```python
from build123d import *

# Parameters (mm, degrees)
SKETCH_1_R      = 1.25
EXTRUDE_1_DEPTH = 2.8
SKETCH_2_R      = 4
SKETCH_2_R_2    = 1.25
EXTRUDE_2_DEPTH = 1.4
SKETCH_3_R      = 1.25
EXTRUDE_3_DEPTH = 2.8
EXTRUDE_4_DEPTH = 3


with BuildPart() as part:
    # 草图1 → 凸台-拉伸1 (new body)
    with BuildSketch(Plane(origin=(0, 0, 0), x_dir=(1, 0, 0), z_dir=(0, 1, 0))):
        with BuildLine():
            Line((0, 5.25), (9.5, 5.25))
            ThreePointArc((9.5, 5.25), (14.75, 0), (9.5, -5.25))
            Line((9.5, -5.25), (0, -5.25))
            ThreePointArc((0, -5.25), (-5.25, 0), (0, 5.25))
        make_face()
        Circle(SKETCH_1_R, mode=Mode.SUBTRACT)
        with Locations((9.5, 0)):
            Circle(SKETCH_1_R, mode=Mode.SUBTRACT)
    extrude(amount=EXTRUDE_1_DEPTH)

    # 草图2 → 凸台-拉伸2 (add)
    with BuildSketch(Plane(origin=(0, 2.8, 0), x_dir=(1, 0, 0), z_dir=(0, 1, 0))):
        Circle(SKETCH_2_R)
        Circle(SKETCH_2_R_2, mode=Mode.SUBTRACT)
        with Locations((9.5, 0)):
            Circle(SKETCH_2_R)
        with Locations((9.5, 0)):
            Circle(SKETCH_2_R_2, mode=Mode.SUBTRACT)
    extrude(amount=EXTRUDE_2_DEPTH)

    # 草图3 → 凸台-拉伸3 (add)
    with BuildSketch(Plane(origin=(0, 4.2, 0), x_dir=(1, 0, 0), z_dir=(0, 1, 0))):
        with BuildLine():
            Line((0, 5.25), (9.5, 5.25))
            ThreePointArc((9.5, 5.25), (14.75, 0), (9.5, -5.25))
            Line((9.5, -5.25), (0, -5.25))
            ThreePointArc((0, -5.25), (-5.25, 0), (0, 5.25))
        make_face()
        Circle(SKETCH_3_R, mode=Mode.SUBTRACT)
        with Locations((9.5, 0)):
            Circle(SKETCH_3_R, mode=Mode.SUBTRACT)
    extrude(amount=EXTRUDE_3_DEPTH)

    # 草图4 → 凸台-拉伸4 (add)
    with BuildSketch(Plane(origin=(0, 0, -5.25), x_dir=(-1, 0, 0), z_dir=(0, 0, -1))):
        with BuildLine():
            ThreePointArc((-1.932304569, 5.576196633), (-4.75, 7), (-7.567695431, 5.576196633))
            Line((-7.567695431, 5.576196633), (-6.360111675, 4.686398076))
            ThreePointArc((-6.360111675, 4.686398076), (-4.75, 5.5), (-3.139888325, 4.686398076))
            Line((-3.139888325, 4.686398076), (-1.932304569, 5.576196633))
        make_face()
        with BuildLine():
            Line((-6.360111675, 2.313601924), (-7.567695431, 1.423803367))
            ThreePointArc((-7.567695431, 1.423803367), (-4.75, 0), (-1.932304569, 1.423803367))
            Line((-1.932304569, 1.423803367), (-3.139888325, 2.313601924))
            ThreePointArc((-3.139888325, 2.313601924), (-4.75, 1.5), (-6.360111675, 2.313601924))
        make_face()
        with BuildLine():
            Line((-6.360111675, 4.686398076), (-7.567695431, 5.576196633))
            ThreePointArc((-7.567695431, 5.576196633), (-8.168041846, 4.252987343), (-8.17928564, 2.8))
            Line((-8.17928564, 2.8), (-6.6234994, 2.8))
            ThreePointArc((-6.6234994, 2.8), (-6.730785439, 3.77656653), (-6.360111675, 4.686398076))
        make_face()
        with BuildLine():
            ThreePointArc((-1.932304569, 1.423803367), (-1.551614092, 2.078617721), (-1.32071436, 2.8))
            Line((-1.32071436, 2.8), (-2.8765006, 2.8))
            ThreePointArc((-2.8765006, 2.8), (-2.99129812, 2.547651483), (-3.139888325, 2.313601924))
            Line((-3.139888325, 2.313601924), (-1.932304569, 1.423803367))
        make_face()
        with BuildLine():
            ThreePointArc((-1.25, 3.5), (-1.424948571, 4.592718169), (-1.932304569, 5.576196633))
            Line((-1.932304569, 5.576196633), (-3.139888325, 4.686398076))
            ThreePointArc((-3.139888325, 4.686398076), (-2.849970612, 4.124410382), (-2.75, 3.5))
            ThreePointArc((-2.75, 3.5), (-2.781879221, 3.144330771), (-2.8765006, 2.8))
            Line((-2.8765006, 2.8), (-1.32071436, 2.8))
            ThreePointArc((-1.32071436, 2.8), (-1.267723464, 3.148218633), (-1.25, 3.5))
        make_face()
        with BuildLine():
            Line((-6.6234994, 2.8), (-8.17928564, 2.8))
            ThreePointArc((-8.17928564, 2.8), (-7.948385908, 2.078617721), (-7.567695431, 1.423803367))
            Line((-7.567695431, 1.423803367), (-6.360111675, 2.313601924))
            ThreePointArc((-6.360111675, 2.313601924), (-6.50870188, 2.547651483), (-6.6234994, 2.8))
        make_face()
    extrude(amount=EXTRUDE_4_DEPTH)


solid = part.part
```
Geometry check sheet. Reference: the model listing, model coordinates, mm. A direction names the side the tool comes from. Coordinates: 2 decimals unless noted, no trailing zeros. Loops run counter-clockwise (first coordinate to the right, second up) from the corner with the lowest first, then second, coordinate; pieces in that order, holes last.
Item 1: Release check for a two-part mould opening along Y. For faces 6 (the face through (5.504, 3.49, -0.176)), 7 (the face through (5, 6, 5.25)), 8 (the face through (5, 7, 0)) record: released by +Y, released by -Y, zero draft, split by the parting line, or undercut.
Item 2: Thickness scan on line 1 (X direction, y = 2, z = 0); line 2 (X direction, y = 3.5, z = 0); line 3 (Y direction, x = 5, z = -4). Record the ranges inside material, lowest first.
Item 3: Access from +Z, -Z, +X, -X, +Y, -Y to the whole of each face (thin tool, end or side, straight path). Record for faces 1 (the face through (7, 4, -5.25)), 2 (the face through (-0.867, 3.49, 3.905)), 3 (the face through (5, 5, -5.25)), 4 (the face through (8, 6, -5.25)), 5 (the face through (1, 6, -5.25)).
Item 4: Sectioned sample at A-A, the plane z = 0. Record the boundary of the cut face in (x, y).
Item 5: Sectioned sample at C-C, the plane y = 3.25. Record the boundary of the cut face in (x, z), then the cut area to 3 significant figures.
Item 6: Go/stop test with flat-tipped pins: pin 1 Ø1 at (y, z) = (4, -2) entering from -X; pin 2 Ø2 at (y, z) = (3.5, 1.5) entering from +X. Record where each tip stops, or that it passes through.
Item 7: Sectioned sample at B-B, the plane z = -6.75. Record the boundary of the cut face in (x, y).
Check result:
1. face 6: undercut
1. face 7: zero draft
1. face 8: released by +Y
2. line 1: x = -5.25 to -1.25, 1.25 to 8.25, 10.75 to 14.75
2. line 2: x = -4 to -1.25, 1.25 to 4, 5.5 to 8.25, 10.75 to 13.5
2. line 3: y = 0 to 2.8, 4.2 to 7
3. face 1: +X, -X
3. face 2: none
3. face 3: -Z
3. face 4: -Z, +X, +Y
3. face 5: -Z, -X, +Y
4. outline: (-5.25, 0) - (-1.25, 0) - (-1.25, 7) - (-5.25, 7) - (-5.25, 4.2) - (-4, 4.2) - (-4, 2.8) - (-5.25, 2.8) - close; (1.25, 0) - (8.25, 0) - (8.25, 7) - (1.25, 7) - close; (10.75, 0) - (14.75, 0) - (14.75, 2.8) - (13.5, 2.8) - (13.5, 4.2) - (14.75, 4.2) - (14.75, 7) - (10.75, 7) - close; hole (4, 2.8) - (5.5, 2.8) - (5.5, 4.2) - (4, 4.2) - close
5. outline: circle Ø8 at (0, 0); (1.26, -8.25) - (2.77, -8.25) - (2.77, -5.25) - (1.26, -5.25) - close; circle Ø8 at (9.5, 0); (6.73, -8.25) - (8.24, -8.25) - (8.24, -5.25) - (6.73, -5.25) - close; hole circle Ø2.5 at (0, 0); hole circle Ø2.5 at (9.5, 0)
5. area: 99.8 mm2
6. pin 1: stops at x = -5.02
6. pin 2: stops at x = 14.69
7. outline: circle Ø7 at (4.75, 3.5); hole circle Ø4 at (4.75, 3.5)
